Read the model definition and answer for the solid it produces. Units are mm, in the model's axes. Face numbers are marked on the shaded views. A direction names the side the tool comes from. Round coordinates to 2 decimals unless told otherwise and drop trailing zeros. Order: outer loops, then holes, each group sorted by start corner. A loop starts at its lowest first (then second) coordinate and runs counter-clockwise, first axis right, second up. Notation, with made-up numbers: (70, 68) - (108, 68) arc R17 ccw to (108, 73) - close; hole circle Ø5 at (6, 47.25). An arc over 180 degrees is marked (long way). Put each result on its own line as item: value. Start each with the question number.
Q1. Section B-B on y = -29.5 is taken. Give the vertices of the cut face in (x, z).
Q2. Section A-A on x = 0 is taken. Give the vertices of the cut face in (y, z), then the cut area to 3 significant figures.
Q3. Section D-D on x = 5 is taken. State how many separate pieces and enclosed holes the cut face has, then the cut area to 3 significant figures.
Q4. For a pull along Y with two mould halves and no side action, classify the marked faces 5, 6 and 7 as pulls with the +Y half, pulls with the -Y half, needs draft (parallel to the pull), parting line crosses it, or undercut.
Q5. Which of the six approach directions +Z, -Z, +X, -X, +Y, -Y give full straight-line access (tool end or side, diameter ignored) to the marked faces 1, 2, 3 and 4?
Q6. Each of these flat-tipped pins is pushed along its axis until it touches: pin 1 Ø0.9 at (y, z) = (-29.5, 4.5) entering from -X; pin 2 Ø1.8 at (x, y) = (5.5, -31) entering from +Z; pin 3 Ø3 at (y, z) = (-31, 19) entering from -X. Where does it stop, or does it pass through?
Q7. Section C-C on z = 15 is taken. Give the vertices of the cut face in (x, y), then the cut area to 3 significant figures.
Q8. Find the intervals of material crossed by line 1 along Z through (x, y) = (2.5, -32.25); line 2 along Z through (x, y) = (-4.25, -33); line 3 along X through (y, z) = (-29.65, 15), in increasing order. Write a range as from..to.
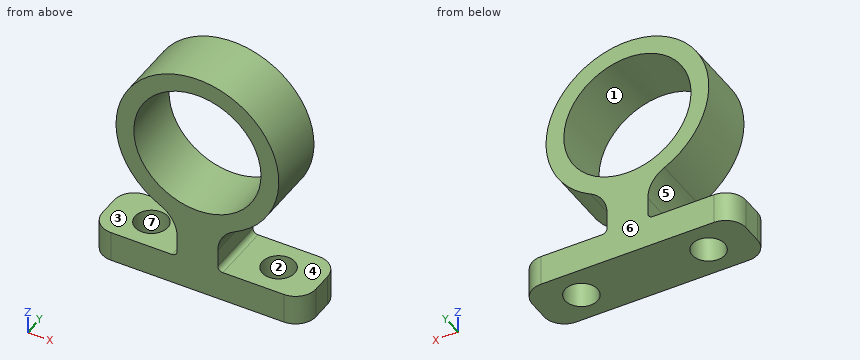
from build123d import *

# Parameters (mm, degrees)
SKETCH_1_W          = 21
SKETCH_1_H          = 6
EXTRUDE_1_DEPTH     = 3
SKETCH_2_R          = 6.25
EXTRUDE_2_DEPTH     = 6
SKETCH_4_R          = 1.6
CUT_EXTRUDE_1_DEPTH = 3
FILLET_1_R          = 0.5
FILLET_2_R          = 3
FILLET_3_R          = 2


with BuildPart() as part:
    # 草图1 → 凸台-拉伸1 (new body)
    with BuildSketch(Plane.XY):
        with Locations((0, -30.20649321)):
            Rectangle(SKETCH_1_W, SKETCH_1_H)
    extrude(amount=EXTRUDE_1_DEPTH)

    # 草图2 → 凸台-拉伸2 (add)
    with BuildSketch(Plane.XZ.offset(33.20649321)):
        with BuildLine():
            ThreePointArc((2, 7.254033308), (0, 23), (-2, 7.254033308))
            Line((-2, 7.254033308), (-2, 3))
            Line((-2, 3), (2, 3))
            Line((2, 3), (2, 7.254033308))
        make_face()
        with Locations(Location((0, 15, 0), (0, 0, 270))):
            Circle(SKETCH_2_R, mode=Mode.SUBTRACT)
    extrude(amount=-EXTRUDE_2_DEPTH)

    # 草图4 → 切除-拉伸1 (cut)
    with BuildSketch(Plane(origin=(0, 0, 0), x_dir=(-1, 0, 0), z_dir=(0, 0, -1))):
        with Locations((-6.25, -30.20649321)):
            Circle(SKETCH_4_R)
        with Locations(Location((6.25, -30.20649321, 0), (0, 0, 180))):
            Circle(SKETCH_4_R)
    extrude(amount=-CUT_EXTRUDE_1_DEPTH, mode=Mode.SUBTRACT)

    # 圆角1
    fillet_1_edges = [part.edges().sort_by_distance(p)[0] for p in [
        (-2, -30.20649321, 3),
        (2, -30.20649321, 3),
    ]]
    fillet(fillet_1_edges, radius=FILLET_1_R)

    # 圆角2
    fillet_2_edges = [part.edges().sort_by_distance(p)[0] for p in [
        (2, -30.20649321, 7.254033308),
        (-2, -30.20649321, 7.254033308),
    ]]
    fillet(fillet_2_edges, radius=FILLET_2_R)

    # 圆角3
    fillet_3_edges = [part.edges().sort_by_distance(p)[0] for p in [
        (10.5, -33.20649321, 1.5),
        (-10.5, -33.20649321, 1.5),
        (-10.5, -27.20649321, 1.5),
        (10.5, -27.20649321, 1.5),
    ]]
    fillet(fillet_3_edges, radius=FILLET_3_R)


solid = part.part
Findings:
1. outline: (-10.5, 0) - (-7.69, 0) - (-7.69, 3) - (-10.5, 3) - close; (-4.81, 0) - (4.81, 0) - (4.81, 3) - (2.5, 3) arc R0.5 cw to (2, 3.5) - (2, 5.2) arc R3 cw to (3.64, 7.87) arc R8 ccw (long way) to (-3.64, 7.87) arc R3 cw to (-2, 5.2) - (-2, 3.5) arc R0.5 cw to (-2.5, 3) - (-4.81, 3) - close; (7.69, 0) - (10.5, 0) - (10.5, 3) - (7.69, 3) - close; hole circle Ø12.5 at (0, 15)
2. outline: (-33.21, 0) - (-27.21, 0) - (-27.21, 8.75) - (-33.21, 8.75) - close; (-33.21, 21.25) - (-27.21, 21.25) - (-27.21, 23) - (-33.21, 23) - close
2. area: 63.0 mm2
3. separate pieces: 4
3. enclosed holes: 0
3. area: 41.9 mm2
4. face 5: needs draft
4. face 6: pulls with the +Y half
4. face 7: undercut
5. face 1: +Y, -Y
5. face 2: -Z
5. face 3: -X, +Y, -Y
5. face 4: +X, +Y, -Y
6. pin 1: x = -2
6. pin 2: z = 21.55
6. pin 3: x = -7.6
7. outline: (-8, -33.21) - (-6.25, -33.21) - (-6.25, -27.21) - (-8, -27.21) - close; (6.25, -33.21) - (8, -33.21) - (8, -27.21) - (6.25, -27.21) - close
7. area: 21.0 mm2
8. line 1: 0..3, 6.86..9.27, 20.73..22.6
8. line 2: 0..3, 8.22..10.42, 19.58..21.78
8. line 3: -8..-6.25, 6.25..8
